Autodesk Inventor part; units mm, degrees
ref_plane "YZ Plane" through (0, 0, 0) normal (1, 0, 0) x (0, 1, 0)
ref_plane "XZ Plane" through (0, 0, 0) normal (0, 1, 0) x (-1, 0, 0)
ref_plane "XY Plane" through (0, 0, 0) normal (0, 0, 1) x (1, 0, 0)
sketch "Sketch1" plane through (0, 0, 0) normal (0, 0, 1) x (1, 0, 0)
  line L0 (0, 0) -> (-98, 0)
  line L1 (-98, 0) -> (-98, 44)
  line L2 (-98, 44) -> (0, 44)
  line L3 (0, 44) -> (0, 0)
  line L4 (5, -5) -> (-103, -5)
  line L5 (-103, -5) -> (-103, 49)
  line L6 (-103, 49) -> (5, 49)
  line L7 (5, 49) -> (5, -5)
  dimension "d0" = 98
  dimension "d1" = 44
  dimension "d2" = 5
  dimension "d3" = 5
  dimension "d4" = 5
  dimension "d5" = 5
extrude "Extrusion1" add sketch "Sketch1" along normal blind 40
sketch "Sketch2" plane through (0, 0, 40) normal (0, 0, 1) x (1, 0, 0)
  line L0 (5, 49) -> (-103, 49)
  line L1 (5, -5) -> (-103, -5)
  line L2 (-103, -5) -> (-103, 49)
  line L3 (-103, 49) -> (5, 49)
  line L4 (5, 49) -> (5, -5)
  line L5 (-93, 34) -> (-10, 34)
  line L6 (-10, 34) -> (-10, 10)
  line L7 (-10, 10) -> (-93, 10)
  line L8 (-93, 10) -> (-93, 34)
  point P0 (0, 0)
  dimension "d10" = 10
  dimension "d11" = 15
  dimension "d12" = 15
  dimension "d13" = 15
extrude "Extrusion2" add sketch "Sketch2" along normal blind 5
sketch "Sketch3" plane through (-103, -5, 0) normal (0, -1, 0) x (1, 0, 0)
  line L0 (108, 0) -> (108, 45)
  line L1 (108, 0) -> (123, 0)
  line L2 (123, 0) -> (123, 15)
  line L3 (123, 15) -> (108, 15)
  line L4 (108, 15) -> (108, 0)
  circle A0 centre (123, 7.5) radius 7.5
  circle A1 centre (123, 7.5) radius 2.5
  line L5 (108, 45) -> (0, 45)
  line L6 (54, 45) -> (54, 61.5977)
  line L7 (0, 0) -> (-15, 0)
  line L8 (-15, 0) -> (-15, 15)
  line L9 (-15, 15) -> (0, 15)
  line L10 (0, 15) -> (0, 0)
  circle A2 centre (-15, 7.5) radius 7.5
  circle A3 centre (-15, 7.5) radius 2.5
  point P0 (103, 0)
  point P1 (5, 0)
  dimension "d14" = 15
  dimension "d15" = 15
  dimension "d16" = 5
extrude "Extrusion3" add sketch "Sketch3" against normal blind 5 contours L0 L3 A0 L1 | A0 L2 A1 | L2 A1 A0 | L7 A2 L9 L10 | A2 L8 A3 | L8 A3 A2
properties part number "PSUBracket"
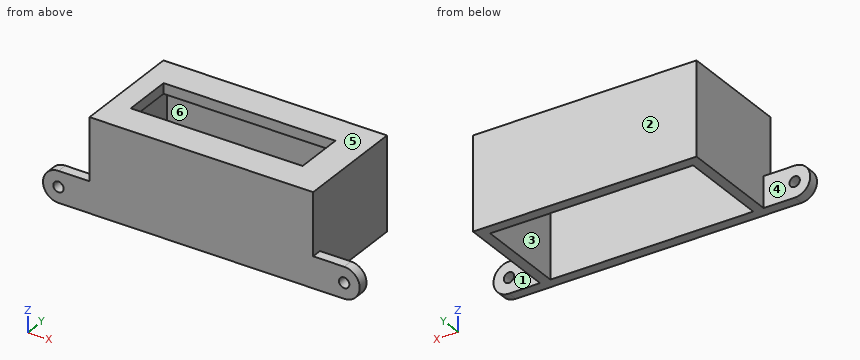
Could you check a few things on this model? Use its own coordinates, in mm. Face numbers are marked on the shaded views. A direction names the side the tool comes from. Give positions to 0.01 mm unless a question says otherwise; leave off trailing zeros. Order: outer loops, then holes, each group sorted by start corner. A loop starts at its lowest first (then second) coordinate and runs counter-clockwise, first axis right, second up.
1. For the marked faces 1, 2, 3 and 4, which set-ups out of +Z, -Z, +X, -X, +Y, -Y let a thin tool reach every point of the face, with its end or its side?
2. We'd pull the mould along X, two halves only. Please class the marked faces 5 and 6: pulls with the +X half, pulls with the -X half, needs draft (parallel to the pull), parting line crosses it, or undercut.
3. Suppose I cut it at A-A (x = -69). List the corners of the cut face in (y, z) for me, plus the area to 3 significant figures.
4. I need wall thicknesses on L1, parallel to X at y = -2.45, z = 7.5; L2, parallel to Z at x = 20, y = -3; L3, parallel to Y at x = -89, z = 7. Which ranges of each line are inside material? Lowest first, please.
5. Will these pins go through, and if not, where does the flat tip stop? P1, Ø4, axis at x = 15, y = -2.5, coming from the +Z side; P2, Ø5.5, axis at y = 16, z = 41.5, coming from the -X side; P3, Ø13, axis at x = -28.5, y = 14.5, coming from the -Z side.
6. Suppose I cut it at B-B (y = 25). List the corners of the cut face in (x, z) for me, plus the area to 3 significant figures.
7. Suppose I cut it at D-D (y = 7). List the corners of the cut face in (x, z) for me, plus the area to 3 significant figures.
8. Suppose I cut it at C-C (z = 7.5). List the corners of the cut face in (x, y) for me.
Solved:
1. face 1: +Z, -Z, +X, +Y
1. face 2: +Z, -Z, +X, -X, +Y
1. face 3: -Z
1. face 4: +Z, -Z, -X, +Y
2. face 5: needs draft
2. face 6: undercut
3. outline: (-5, 0) - (0, 0) - (0, 40) - (10, 40) - (10, 45) - (-5, 45) - close; (34, 40) - (44, 40) - (44, 0) - (49, 0) - (49, 45) - (34, 45) - close
3. area: 550 mm2
4. L1: x = -125.5 to -120.5, -115.5 to 17.5, 22.5 to 27.5
4. L2: z = 0 to 5, 10 to 15
4. L3: y = -5 to 0, 44 to 49
5. P1: stops at z = 15
5. P2: stops at x = -103
5. P3: stops at z = 40
6. outline: (-103, 0) - (-98, 0) - (-98, 40) - (-93, 40) - (-93, 45) - (-103, 45) - close; (-10, 40) - (0, 40) - (0, 0) - (5, 0) - (5, 45) - (-10, 45) - close
6. area: 525 mm2
7. outline: (-103, 0) - (-98, 0) - (-98, 40) - (0, 40) - (0, 0) - (5, 0) - (5, 45) - (-103, 45) - close
7. area: 940 mm2
8. outline: (-125.5, -5) - (-120.5, -5) - (-120.5, 0) - (-125.5, 0) - close; (-115.5, -5) - (17.5, -5) - (17.5, 0) - (5, 0) - (5, 49) - (-103, 49) - (-103, 0) - (-115.5, 0) - close; (22.5, -5) - (27.5, -5) - (27.5, 0) - (22.5, 0) - close; hole (-98, 0) - (0, 0) - (0, 44) - (-98, 44) - close
